```python
from build123d import *

# Parameters (mm, degrees)
SKETCH1_R               = 9
BOSS_EXTRUDE1_DEPTH     = 6
SKETCH3_R               = 5.5
CUT_EXTRUDE2_DEPTH      = 1
CUT_EXTRUDE2_DEPTH_BACK = 7
CUT_EXTRUDE3_REACH      = 8
SKETCH6_R               = 2.5


with BuildPart() as part:
    # Sketch1 → Boss-Extrude1 (new body)
    with BuildSketch(Plane(origin=(0, 0, 0), x_dir=(1, 0, 0), z_dir=(0, 1, 0))):
        with BuildLine():
            Line((-50, -65), (50, -65))
            ThreePointArc((50, -65), (60.606601718, -60.606601718), (65, -50))
            Line((65, -50), (65, 50))
            ThreePointArc((65, 50), (60.606601718, 60.606601718), (50, 65))
            Line((50, 65), (-50, 65))
            ThreePointArc((-50, 65), (-60.606601718, 60.606601718), (-65, 50))
            Line((-65, 50), (-65, -50))
            ThreePointArc((-65, -50), (-60.606601718, -60.606601718), (-50, -65))
        make_face()
        Circle(SKETCH1_R, mode=Mode.SUBTRACT)
    extrude(amount=BOSS_EXTRUDE1_DEPTH)

    # Sketch3 → Cut-Extrude2 (cut, two sides)
    with BuildSketch(Plane(origin=(0, 6, 0), x_dir=(1, 0, 0), z_dir=(0, 1, 0))) as cut_extrude2_sk:
        with Locations((-50, 50)):
            Circle(SKETCH3_R)
        with Locations((50, 50)):
            Circle(SKETCH3_R)
        with Locations((50, -50)):
            Circle(SKETCH3_R)
        with Locations((-50, -50)):
            Circle(SKETCH3_R)
    extrude(amount=CUT_EXTRUDE2_DEPTH, mode=Mode.SUBTRACT)
    extrude(cut_extrude2_sk.sketch, amount=-CUT_EXTRUDE2_DEPTH_BACK, mode=Mode.SUBTRACT)

    # Sketch6 → Cut-Extrude3 (cut, up to next)
    with BuildSketch(Plane(origin=(0, 6, 0), x_dir=(1, 0, 0), z_dir=(0, 1, 0)), mode=Mode.PRIVATE) as cut_extrude3_sk1:
        with Locations((33, 48)):
            Circle(SKETCH6_R)
    cut_extrude3_tool1 = extrude(cut_extrude3_sk1.sketch, amount=-CUT_EXTRUDE3_REACH, mode=Mode.PRIVATE) & part.part
    add(cut_extrude3_tool1.solids().sort_by_distance((33, 6, -48))[0], mode=Mode.SUBTRACT)
    # Sketch6 → Cut-Extrude3 (cut, up to next)
    with BuildSketch(Plane(origin=(0, 6, 0), x_dir=(1, 0, 0), z_dir=(0, 1, 0)), mode=Mode.PRIVATE) as cut_extrude3_sk2:
        with Locations((33, -18)):
            Circle(SKETCH6_R)
    cut_extrude3_tool2 = extrude(cut_extrude3_sk2.sketch, amount=-CUT_EXTRUDE3_REACH, mode=Mode.PRIVATE) & part.part
    add(cut_extrude3_tool2.solids().sort_by_distance((33, 6, 18))[0], mode=Mode.SUBTRACT)
    # Sketch6 → Cut-Extrude3 (cut, up to next)
    with BuildSketch(Plane(origin=(0, 6, 0), x_dir=(1, 0, 0), z_dir=(0, 1, 0)), mode=Mode.PRIVATE) as cut_extrude3_sk3:
        with Locations((-33, 48)):
            Circle(SKETCH6_R)
    cut_extrude3_tool3 = extrude(cut_extrude3_sk3.sketch, amount=-CUT_EXTRUDE3_REACH, mode=Mode.PRIVATE) & part.part
    add(cut_extrude3_tool3.solids().sort_by_distance((-33, 6, -48))[0], mode=Mode.SUBTRACT)
    # Sketch6 → Cut-Extrude3 (cut, up to next)
    with BuildSketch(Plane(origin=(0, 6, 0), x_dir=(1, 0, 0), z_dir=(0, 1, 0)), mode=Mode.PRIVATE) as cut_extrude3_sk4:
        with Locations((-33, -18)):
            Circle(SKETCH6_R)
    cut_extrude3_tool4 = extrude(cut_extrude3_sk4.sketch, amount=-CUT_EXTRUDE3_REACH, mode=Mode.PRIVATE) & part.part
    add(cut_extrude3_tool4.solids().sort_by_distance((-33, 6, 18))[0], mode=Mode.SUBTRACT)


solid = part.part
```
Here's how the part is built. I have some questions about the finished solid (model axes, mm). Give positions to 0.01 mm unless a question says otherwise; leave off trailing zeros. Loops run counter-clockwise (first coordinate to the right, second up) from the corner with the lowest first, then second, coordinate; pieces in that order, holes last. Notation, with made-up numbers: (62, 50.25) -> (89, 50.25) arc R19 cw to (89, 85.25) -> close; hole circle Ø2 at (55, 56.25). An arc over 180 degrees is marked (long way). Use one line per item in the form item = value. Start each with the question number.
1) Imagine slicing it at D-D (x = -3.5). Please give me the cut outline in (y, z).
2) Imagine slicing it at B-B (y = 1.45). Count the separate pieces of the cut face and the enclosed holes in it, then the cut area to 3 significant figures.
3) Please list where these lines run through material, in increasing order: line 1 along Z through (x, y) = (-50, 2.75); line 2 along X through (y, z) = (1, 47).
4) Imagine slicing it at C-C (z = 18). Please give me the cut outline in (x, y).
5) Thinking about a two-plate mould opening in Z: for faces 1 (the face through (60.72, 2.96, -60.49)), 2 (the face through (60.49, 2.96, 60.72)), 3 (the face through (32.46, 3.04, -45.56)), 4 (the face through (-35.5, 3, 17.9)), which applies, +Z half, -Z half, draft (parallel to the pull), parting line (faces both ways), or undercut?
6) Imagine slicing it at A-A (z = 0). Please give me the cut outline in (x, y).
Check values:
q1.outline = (0, -65) -> (6, -65) -> (6, -8.29) -> (0, -8.29) -> close; (0, 8.29) -> (6, 8.29) -> (6, 65) -> (0, 65) -> close
q2.separate_pieces = 1
q2.enclosed_holes = 9
q2.area = 16,000 mm^2
q3.line_1 = -65 to -55.5, -44.5 to 44.5, 55.5 to 65
q3.line_2 = -65 to -54.61, -45.39 to 45.39, 54.61 to 65
q4.outline = (-65, 0) -> (-35.5, 0) -> (-35.5, 6) -> (-65, 6) -> close; (-30.5, 0) -> (30.5, 0) -> (30.5, 6) -> (-30.5, 6) -> close; (35.5, 0) -> (65, 0) -> (65, 6) -> (35.5, 6) -> close
q5.face_1 = -Z half
q5.face_2 = +Z half
q5.face_3 = undercut
q5.face_4 = undercut
q6.outline = (-65, 0) -> (-9, 0) -> (-9, 6) -> (-65, 6) -> close; (9, 0) -> (65, 0) -> (65, 6) -> (9, 6) -> close
